from build123d import *

# Parameters (mm, degrees)
SKETCH_1_W          = 5
SKETCH_1_H          = 3.9
EXTRUDE_1_DEPTH     = 12.8
SKETCH_2_R          = 1
CUT_EXTRUDE_1_DEPTH = 5
SKETCH_3_W          = 1.5
SKETCH_3_H          = 7.9
EXTRUDE_2_DEPTH     = 5
SKETCH_4_R          = 1.1
CUT_EXTRUDE_2_DEPTH = 5
FILLET_1_R          = 3
FILLET_2_R          = 3
FILLET_3_R          = 1


with BuildPart() as part:
    # 草图1 → 凸台-拉伸1 (new body)
    with BuildSketch(Plane.XY):
        Rectangle(SKETCH_1_W, SKETCH_1_H)
    extrude(amount=EXTRUDE_1_DEPTH)

    # 草图2 → 切除-拉伸1 (cut)
    with BuildSketch(Plane(origin=(0, 0, 0), x_dir=(-1, 0, 0), z_dir=(0, 0, -1))):
        with Locations((0, -0.05)):
            Circle(SKETCH_2_R)
    extrude(amount=-CUT_EXTRUDE_1_DEPTH, mode=Mode.SUBTRACT)

    # 草图3 → 凸台-拉伸2 (add)
    with BuildSketch(Plane.XY.offset(12.8)):
        with Locations((1.75, 2)):
            Rectangle(SKETCH_3_W, SKETCH_3_H)
        with Locations((-1.75, 2)):
            Rectangle(SKETCH_3_W, SKETCH_3_H)
    extrude(amount=EXTRUDE_2_DEPTH)

    # 草图4 → 切除-拉伸2 (cut)
    with BuildSketch(Plane(origin=(2.5, 0, 0), x_dir=(0, 0, -1), z_dir=(1, 0, 0))):
        with Locations(Location((-15.3, 0.55, 0), (0, 0, 90))):
            Circle(SKETCH_4_R)
    extrude(amount=-CUT_EXTRUDE_2_DEPTH, mode=Mode.SUBTRACT)

    # 圆角1
    # the kernel refuses this fillet: 3 mm, written as the material it takes off along each edge
    with BuildSketch(Plane(origin=(-2.5, -1.95, -7.5), x_dir=(0, 1, 0), z_dir=(0, 0, 1)), Plane(origin=(2.5, -1.95, 25.3), x_dir=(0, 1, 0), z_dir=(0, 0, -1))) as fillet_1_piece_1:
        with BuildLine():
            CenterArc((FILLET_1_R, -FILLET_1_R), FILLET_1_R, 90, 90)
            Line((0, -FILLET_1_R), (0, 0))
            Line((0, 0), (FILLET_1_R, 0))
        make_face()
    extrude(amount=32.8, mode=Mode.SUBTRACT)

    # 圆角2
    # the kernel refuses this fillet: 3 mm, written as the material it takes off along each edge
    with BuildSketch(Plane(origin=(2.5, 5.95, 6.304809472), x_dir=(0, -1, 0), z_dir=(0, 0, 1))) as fillet_2_piece_1:
        with BuildLine():
            CenterArc((2.598076211, -3), FILLET_2_R, 90, 60)
            Line((0, -1.5), (-0.051961524, -1.47))
            ThreePointArc((-0.051961524, -1.47), (-0.06, -0.75), (-0.06, 0))
            Line((-0.06, 0), (0, 0.06))
            Line((0, 0.06), (2.598076211, 0.06))
            Line((2.598076211, 0.06), (2.598076211, 0))
        make_face()
    extrude(amount=17.990381057, mode=Mode.SUBTRACT)
    with BuildSketch(Plane(origin=(-2.5, 5.95, 6.304809472), x_dir=(0, -1, 0), z_dir=(0, 0, 1))) as fillet_2_piece_2:
        with BuildLine():
            CenterArc((2.598076211, 3), FILLET_2_R, 210, 60)
            Line((0, 1.5), (-0.051961524, 1.47))
            ThreePointArc((-0.051961524, 1.47), (-0.06, 0.75), (-0.06, 0))
            Line((-0.06, 0), (0, -0.06))
            Line((0, -0.06), (2.598076211, -0.06))
            Line((2.598076211, -0.06), (2.598076211, 0))
        make_face()
    extrude(amount=17.990381057, mode=Mode.SUBTRACT)

    # 圆角3
    fillet_3_edges = [part.edges().sort_by_distance(p)[0] for p in [
        (-2.098076211, -0.45, 17.8),
        (2.5, 2.200961894, 17.8),
        (2.098076211, -0.45, 17.8),
        (2.098076211, 4.851923789, 17.8),
        (-2.5, 2.200961894, 17.8),
        (-2.098076211, 4.851923789, 17.8),
    ]]
    fillet(fillet_3_edges, radius=FILLET_3_R)


solid = part.part
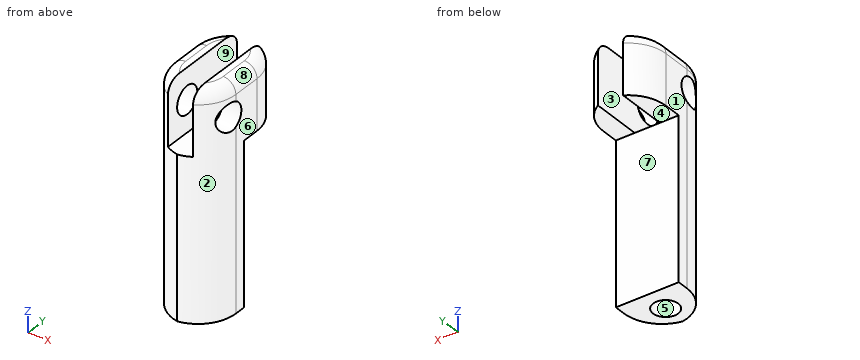
Here's how the part is built. I have some questions about the finished solid (model axes, mm). Face numbers are marked on the shaded views. A direction names the side the tool comes from. Give positions to 0.01 mm unless a question says otherwise; leave off trailing zeros. Order: outer loops, then holes, each group sorted by start corner. A loop starts at its lowest first (then second) coordinate and runs counter-clockwise, first axis right, second up. Notation, with made-up numbers: (-25.75, -7.5) -> (-11.75, -7.5) arc R12 cw to (-11.75, 4.5) -> close; hole circle Ø8 at (15, 22.5). An arc over 180 degrees is marked (long way). Use a Markdown table: item, result. Add a question column.
Item 1: Imagine slicing it at B-B on z = 14. Please give me the cut outline in (x, y), plus the area to 3 significant figures.
Item 2: If we mould it in two halves opening along X, with no side actions, what happens to the marked faces 1, 2, 3 and 4? For each: pulls with the +X half, pulls with the -X half, needs draft (parallel to the pull), parting line crosses it, or undercut.
Item 3: Imagine slicing it at D-D on z = 7.75. Please give me the cut outline in (x, y).
Item 4: Will these pins go through, and if not, where does the flat tip stop? pin 1 (0.6 mm diameter, centred on x = -0.5, y = -0.5, fed in from +Z); pin 2 (4 mm diameter, centred on y = 3.5, z = 12.5, fed in from -X); pin 3 (1.2 mm diameter, centred on x = 1.5, y = 3.5, fed in from -Z); pin 4 (1.8 mm diameter, centred on x = 0, y = -0.05, fed in from -Z).
Item 5: I need wall thicknesses on line 1 (X direction, y = 2.75, z = 16); line 2 (Z direction, x = -1.95, y = 0.55); line 3 (Z direction, x = 0.3, y = -1.5). Which ranges of each line are inside material? Lowest first, please.
Item 6: Imagine slicing it at C-C on x = 0.75. Please give me the cut outline in (y, z).
Item 7: For the marked faces 5, 6, 7, 8 and 9, which set-ups out of +Z, -Z, +X, -X, +Y, -Y let a thin tool reach every point of the face, with its end or its side?
Item 8: Imagine slicing it at A-A on y = 2.25. Please give me the cut outline in (x, z).
Data:
| question | item | result |
|---|---|---|
| 1 | outline | (-2.5, 1.05) arc R3 ccw to (-1, -1.55) -> (-1, 5.95) arc R3 ccw to (-2.5, 3.35) -> close; (1, -1.55) arc R3 ccw to (2.5, 1.05) -> (2.5, 3.35) arc R3 ccw to (1, 5.95) -> close |
| 1 | area | 18.0 mm² |
| 2 | face 1 | pulls with the -X half |
| 2 | face 2 | pulls with the +X half |
| 2 | face 3 | undercut |
| 2 | face 4 | needs draft |
| 3 | outline | (-2.5, 1.05) arc R3 ccw to (0, -1.91) arc R3 ccw to (2.5, 1.05) -> (2.5, 1.95) -> (-2.5, 1.95) -> close |
| 4 | pin 1 | stops at z = 12.8 |
| 4 | pin 2 | stops at x = -2.5 |
| 4 | pin 3 | stops at z = 12.8 |
| 4 | pin 4 | stops at z = 5 |
| 5 | line 1 | x = -2.5 to -1, 1 to 2.5 |
| 5 | line 2 | z = 0 to 14.2, 16.4 to 17.67 |
| 5 | line 3 | z = 0 to 12.8 |
| 6 | outline | (-1.68, 0) -> (-0.71, 0) -> (-0.71, 5) -> (0.61, 5) -> (0.61, 0) -> (1.95, 0) -> (1.95, 12.8) -> (-1.68, 12.8) -> close |
| 7 | face 5 | -Z |
| 7 | face 6 | +Z, -Z, +X, +Y, -Y |
| 7 | face 7 | -Z, +X, -X, +Y |
| 7 | face 8 | +Z, +X, +Y, -Y |
| 7 | face 9 | +Z, +Y, -Y |
| 8 | outline | (-2.5, 12.8) -> (-1, 12.8) -> (-1, 17.8) -> (-1.5, 17.8) arc R1 ccw to (-2.5, 16.8) -> close; (1, 12.8) -> (2.5, 12.8) -> (2.5, 16.8) arc R1 ccw to (1.5, 17.8) -> (1, 17.8) -> close |
